from build123d import *


with BuildPart() as part:
    # Esboço5 → Revolução1 (revolve)
    with BuildSketch(Plane(origin=(0, 0, 0), x_dir=(0, 0, -1), z_dir=(1, 0, 0))):
        with BuildLine():
            Line((-4, 28), (6, 28))
            Line((6, 28), (6, -28))
            Line((6, -28), (1.752133554, -28))
            Line((1.752133554, -28), (1.752133554, -4))
            Line((1.752133554, -4), (-2.370874425, -4))
            Line((-2.370874425, -4), (-2.370874425, 0))
            ThreePointArc((-2.370874425, 0), (0.180241373, 1.421453775), (0.313828383, 4.338794544))
            Line((0.313828383, 4.338794544), (-6, 17))
            Line((-6, 17), (-6, 26))
            Line((-6, 26), (-4, 28))
        make_face()
    revolve(axis=Axis((0, 28, 4), (0, -0.7071067811865436, 0.7071067811865516)))


solid = part.part
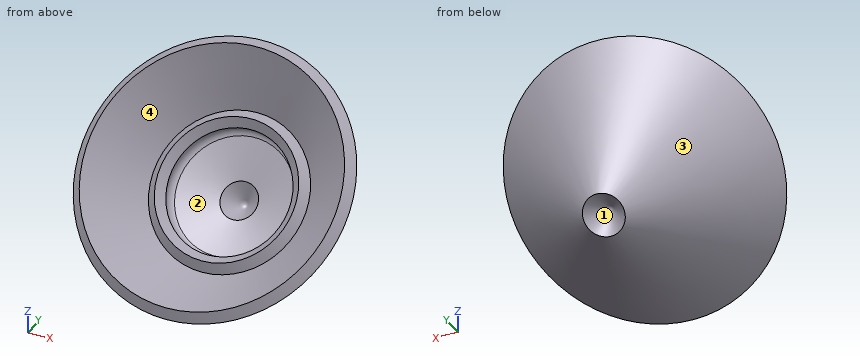
Geometry: final body of the model. Coordinates: model frame, mm. Face numbers are marked on the shaded views. A direction names the side the tool comes from. Give positions to 0.01 mm unless a question says otherwise; leave off trailing zeros. Answer as a JSON object with one key per item and string values.
1. Access query for the marked faces 1 and 2. Directions: +Z, -Z, +X, -X, +Y, -Y. A direction counts if a zero-diameter tool reaches every point of the face in a straight line with its end or side. Return the directions, or none.
Ans:
{"face 1": "-Z, +Y", "face 2": "none"}
2. Ray query, probe 1 along X at (y, z) = (13.5, 17); probe 2 along X at (y, z) = (7, 27.5); probe 3 along Y at (x, z) = (14, 16.5). Return the intervals inside material, ascending. Write a range as from..to.
Ans:
{"probe 1": "x = -33.57..-27.56, -25.79..-21.72, 21.72..25.79, 27.56..33.57", "probe 2": "x = -45.57..-39.56, 39.56..45.57", "probe 3": "y = 23.38..33.64"}
3. Mould query, pull axis X, two halves, no side actions, for the marked faces 3 and 4. Classes: pulls with the +X half, pulls with the -X half, needs draft (parallel to the pull), parting line crosses it, or undercut.
Ans:
{"face 3": "parting line crosses it", "face 4": "undercut"}
4. Contact query for flat-ended pins moving along their axis: pin 1 (10 mm diameter, centred on y = 24.5, z = 51, fed in from -X); pin 2 (10 mm diameter, centred on y = 7.5, z = 28, fed in from +X); pin 3 (4 mm diameter, centred on x = 9, y = -0.5, fed in from +Z). Output: stop coordinate, or through.
Ans:
{"pin 1": "stops at x = -38.13", "pin 2": "stops at x = 46.67", "pin 3": "stops at z = 4.39"}
